```python
from build123d import *

# Parameters (mm, degrees)
F0_R     = 200
F0_R_2   = 10
F1_DEPTH = 20


# Not quite as in the source:
# - a feature names something its author has since deleted; it is built from what else it names


with BuildPart() as f1:
    # F0 (on Top) → F1 (new body)
    with BuildSketch(Plane.XY):
        Circle(F0_R)
        with Locations((-53.5756805311, -129.3431345516)):
            Circle(F0_R_2, mode=Mode.SUBTRACT)
        with Locations((-129.3431345516, -53.5756805311)):
            Circle(F0_R_2, mode=Mode.SUBTRACT)
        with Locations((53.5756805311, -129.3431345516)):
            Circle(F0_R_2, mode=Mode.SUBTRACT)
        with Locations((129.3431345516, -53.5756805311)):
            Circle(F0_R_2, mode=Mode.SUBTRACT)
        with Locations((-129.3431345516, 53.5756805311)):
            Circle(F0_R_2, mode=Mode.SUBTRACT)
        with Locations((-53.5756805311, 129.3431345516)):
            Circle(F0_R_2, mode=Mode.SUBTRACT)
        with Locations((129.3431345516, 53.5756805311)):
            Circle(F0_R_2, mode=Mode.SUBTRACT)
        with BuildLine():
            ThreePointArc((49.7488462075, 120.1043392265), (48.0199782009, 137.6578306746), (63.5756805311, 129.3431345516))
            ThreePointArc((63.5756805311, 129.3431345516), (59.1313828613, 121.0284384286), (49.7488462075, 120.1043392265))
        make_face(mode=Mode.SUBTRACT)
    extrude(amount=F1_DEPTH)


solid = f1.part
```
Geometry check sheet. Reference: the model listing, model coordinates, mm. Coordinates: 2 decimals unless noted, no trailing zeros. Loops run counter-clockwise (first coordinate to the right, second up) from the corner with the lowest first, then second, coordinate; pieces in that order, holes last. Notation, with made-up numbers: (46, 85.5) - (64, 85.5) arc R13 ccw to (64, 101.5) - close; hole circle Ø9 at (63, 76). An arc over 180 degrees is marked (long way). One line per item, written item: value. Start each with the question number.
(1) Mould release check, pull along Y, two halves, no side actions. Record for faces 1 (the cylindrical face through (138.581, 49.746, 9.86)), 2 (the flat face through (-3, 3, 0)), 3 (the cylindrical face through (190.764, 60.075, 9.86)), 4 (the cylindrical face through (63, -126, 10)): released by +Y, released by -Y, zero draft, split by the parting line, or undercut.
(2) Cross-section at D-D on x = 95. Enter the section's corners in (y, z).
(3) Material ranges on line 1 (X direction, y = 136.5, z = 11); line 2 (Y direction, x = -51, z = 7.25); line 3 (Y direction, x = 52, z = 1.5), recorded low to high. Write a range as [from, to].
(4) Cross-section at C-C on y = 96.5. Enter the section's corners in (x, z).
(5) Cross-section at B-B on z = 12.25. Count the separate pieces of the cut face and the enclosed holes in it, plus the area to 3 significant figures.
(6) Depth check by flat-ended pin: P1, Ø23, axis at x = -129.34, y = 53.58, coming from the +Z side; P2, Ø18, axis at x = 129.34, y = 53.58, coming from the -Z side; P3, Ø3, axis at x = 30.5, z = 9.5, coming from the -Y side; P4, Ø6, axis at x = 30.5, z = 15, coming from the +Y side. Enter the tip coordinate at first touch or a pass-through.
(7) Cross-section at A-A on x = -130. Enter the section's corners in (y, z), plus the area to 3 significant figures.
Results below:
1. face 1: undercut
1. face 2: zero draft
1. face 3: split by the parting line
1. face 4: undercut
2. outline: (-176, 0) - (176, 0) - (176, 20) - (-176, 20) - close
3. line 1: x = [-146.18, -60.56], [-46.59, 46.59], [60.56, 146.18]
3. line 2: y = [-193.39, -139.01], [-119.68, 119.68], [139.01, 193.39]
3. line 3: y = [-193.12, -139.22], [-119.47, 119.47], [139.22, 193.12]
4. outline: (-175.18, 0) - (175.18, 0) - (175.18, 20) - (-175.18, 20) - close
5. separate pieces: 1
5. enclosed holes: 8
5. area: 123,000 mm2
6. P1: stops at z = 20
6. P2: passes through
6. P3: stops at y = -197.89
6. P4: stops at y = 198.1
7. outline: (-151.99, 0) - (-63.55, 0) - (-63.55, 20) - (-151.99, 20) - close; (-43.6, 0) - (43.6, 0) - (43.6, 20) - (-43.6, 20) - close; (63.55, 0) - (151.99, 0) - (151.99, 20) - (63.55, 20) - close
7. area: 5,280 mm2
